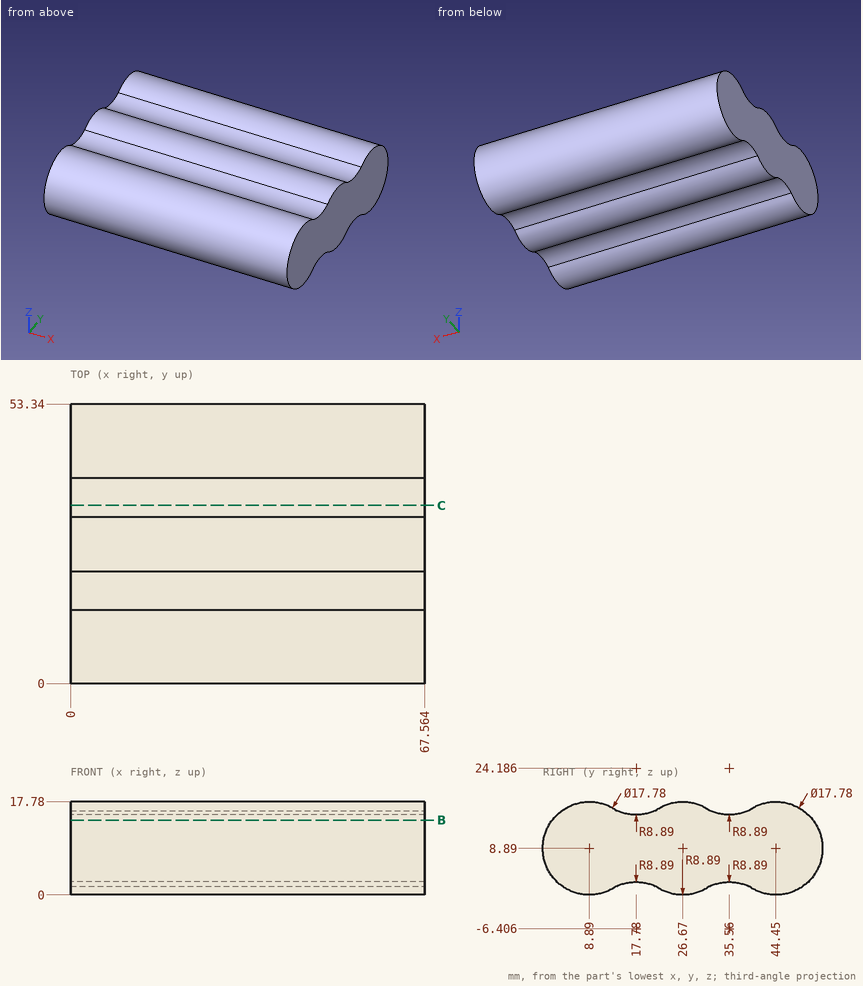
For this review, use the dimensioned drawing (mm, ordinates from the lowest corner) and the shaded views. Give positions to 0.01 mm unless a question says otherwise; leave off trailing zeros. Order: outer loops, then holes, each group sorted by start corner. A loop starts at its lowest first (then second) coordinate and runs counter-clockwise, first axis right, second up. Notation, with made-up numbers: M 82.25,13 L 88.25,13 A6 ccw 88.25,20 Z; hole C 83.5,48.25 d2. An arc over 180 degrees is marked long. Use one line per item in the form item = value. Start each with the question number.
Item 1: Insertion check: pin 1 Ø3 at (x, y) = (52.5, 35.5) entering from +Z (1 decimal); pin 2 Ø2 at (x, y) = (17.5, 28) entering from +Z; pin 3 Ø8 at (x, y) = (25.5, 34.5) entering from -Z. Each pin has a flat end and moves straight along its axis. Give the tip position at first contact, or say it passes through.
Item 2: To check wall thickness, follow line 1 along Y through (x, z) = (24.5, 16.25) (1 decimal); line 2 along Z through (x, y) = (42, 44); line 3 along Z through (x, y) = (43, 2) (1 decimal). State the ranges of each line that lie inside material, in increasing order. Write a range as from..to.
Item 3: We need section C-C on y = 34. Give the boundary of the cut face in (x, z) (1 decimal), plus the area to 3 significant figures.
Item 4: We need section B-B on z = 14.25. Give the boundary of the cut face in (x, y).
Completed:
q1.pin_1 = 15.4
q1.pin_2 = 17.77
q1.pin_3 = 0.87
q2.line_1 = 3.9..13.9, 21.7..31.7, 39.5..49.4
q2.line_2 = 0.01..17.77
q2.line_3 = 3.3..14.5
q3.outline = M 0,2.3 L 67.6,2.3 L 67.6,15.4 L 0,15.4 Z
q3.area = 884 mm²
q4.outline = M 0,1.8 L 67.56,1.8 L 67.56,51.54 L 0,51.54 Z
